Verification items for the finished model (mm, model axes). Give positions to 0.01 mm unless a question says otherwise; leave off trailing zeros. Order: outer loops, then holes, each group sorted by start corner. A loop starts at its lowest first (then second) coordinate and runs counter-clockwise, first axis right, second up. Notation, with made-up numbers: (-35, -25) -> (-15, -25) arc R17 cw to (-15, -16) -> close; hole circle Ø11 at (27.5, -10.75). An arc over 180 degrees is marked (long way). Return JSON: item names as keys, results as strings. Group by question number.
(1) Release check for a two-part mould opening along Z. For faces 1 (the face through (0, 23, 2)), 2 (the face through (0.867, 22.192, 3.905)), 3 (the face through (-2, 0, -2)) record: pulls with the +Z half, pulls with the -Z half, needs draft (parallel to the pull), parting line crosses it, or undercut.
(2) Cross-section at B-B on y = 38. Enter the section's corners in (x, z), then the cut area to 3 significant figures.
(3) Depth check by flat-ended pin: pin 1 Ø1 at (x, y) = (-2, 18) entering from +Z. Enter the tip coordinate at first touch or a pass-through.
(4) Thickness scan on line 1 along Z through (x, y) = (0, 35); line 2 along Z through (x, y) = (0.5, 13.5); line 3 along X through (y, z) = (36, 1.5). Record the ranges inside material, lowest first.
(5) Cross-section at A-A on x = 0. Enter the section's corners in (y, z).
Autodesk Inventor part; units mm, degrees
ref_plane "YZ Plane" through (0, 0, 0) normal (1, 0, 0) x (0, 1, 0)
ref_plane "XZ Plane" through (0, 0, 0) normal (0, 1, 0) x (-1, 0, 0)
ref_plane "XY Plane" through (0, 0, 0) normal (0, 0, 1) x (1, 0, 0)
sketch "Sketch1" plane through (0, 0, 0) normal (0, 1, 0) x (-1, 0, 0)
  circle A0 centre (0, 0) radius 4
  dimension "d0" = 8
extrude "Extrusion1" add sketch "Sketch1" along normal blind 45
chamfer "Chamfer1" distance 0.5 angle 45 2 edges at (4, 45, 0) (4, 0, 0)
sketch "Sketch2" plane through (0, 45, 0) normal (0, 1, 0) x (1, 0, 0)
  circle A0 centre (0, 0) radius 2
  dimension "d6" = 4
extrude "Extrusion2" cut sketch "Sketch2" against normal blind 45
properties part number "pin_8_45"
Verdict:
{
 "1": {"face 1": "undercut", "face 2": "parting line crosses it", "face 3": "needs draft"},
 "2": {"outline": "circle Ø8 at (0, 0); hole circle Ø4 at (0, 0)", "area": "37.7 mm²"},
 "3": {"pin 1": "z = 3.71"},
 "4": {"line 1": "-4 to -2, 2 to 4", "line 2": "-3.97 to -1.94, 1.94 to 3.97", "line 3": "-3.71 to -1.32, 1.32 to 3.71"},
 "5": {"outline": "(0, -3.5) -> (0.5, -4) -> (44.5, -4) -> (45, -3.5) -> (45, -2) -> (0, -2) -> close; (0, 2) -> (45, 2) -> (45, 3.5) -> (44.5, 4) -> (0.5, 4) -> (0, 3.5) -> close"}
}
